Input: part model. Units: mm. Frame: model coordinates. Round coordinates to 2 decimals unless told otherwise and drop trailing zeros. Order: outer loops, then holes, each group sorted by start corner. A loop starts at its lowest first (then second) coordinate and runs counter-clockwise, first axis right, second up.
Item 1: Cut plane A-A on y = 4.3. Give the number of separate pieces and of enclosed holes in the cut face, then the cut area to 3 significant figures.
Item 2: Line query: L1, parallel to X at y = 3.5, z = -2.5 (3 decimals); L2, parallel to Y at x = 0, z = 1.75; L3, parallel to Y at x = 27, z = -3. Output: solid intervals per line, ascending.
Item 3: Cut plane D-D on x = 34.5. Output: boundary loops of the cut face in (y, z), then the cut area to 3 significant figures.
Item 4: First-contact query: pin 1 (1 mm diameter, centred on x = -6.5, z = 3.5, fed in from +Y); pin 2 (1.5 mm diameter, centred on x = -19, y = 3.5, fed in from -Z). Flat tips, straight axial feed; report the tip coordinate or a pass-through.
Item 5: Cut plane B-B on x = 9. Output: boundary loops of the cut face in (y, z), then the cut area to 3 significant figures.
Item 6: Cut plane C-C on z = 1.25. Output: boundary loops of the cut face in (x, y).
```python
from build123d import *

# Parameters (mm, degrees)
SKETCH1_W           = 43.1
SKETCH1_H           = 8
BOSS_EXTRUDE1_DEPTH = 2
SKETCH2_W           = 10
SKETCH2_H           = 2
BOSS_EXTRUDE2_DEPTH = 3
SKETCH3_W           = 33.1
SKETCH3_H           = 2
BOSS_EXTRUDE3_DEPTH = 1
CUT_EXTRUDE1_DEPTH  = 45.120403443


with BuildPart() as part:
    # Sketch1 → Boss-Extrude1 (new body)
    with BuildSketch(Plane(origin=(0, 0, 0), x_dir=(1, 0, 0), z_dir=(0, 1, 0))):
        with Locations((21.55, 0)):
            Rectangle(SKETCH1_W, SKETCH1_H)
    boss_extrude1 = extrude(amount=BOSS_EXTRUDE1_DEPTH)

    # Sketch2 → Boss-Extrude2 (add)
    with BuildSketch(Plane(origin=(0, 2, 0), x_dir=(1, 0, 0), z_dir=(0, 1, 0))):
        with Locations((38.1, -3)):
            Rectangle(SKETCH2_W, SKETCH2_H)
        with Locations((38.1, 3)):
            Rectangle(SKETCH2_W, SKETCH2_H)
    boss_extrude2 = extrude(amount=BOSS_EXTRUDE2_DEPTH)

    # Sketch3 → Boss-Extrude3 (add)
    with BuildSketch(Plane(origin=(0, 2, 0), x_dir=(1, 0, 0), z_dir=(0, 1, 0))):
        with Locations((16.55, -3)):
            Rectangle(SKETCH3_W, SKETCH3_H)
        with Locations((16.55, 3)):
            Rectangle(SKETCH3_W, SKETCH3_H)
    boss_extrude3 = extrude(amount=BOSS_EXTRUDE3_DEPTH)

    # Sketch4 → Cut-Extrude1 (cut, through all)
    with BuildSketch(Plane.XY.offset(4)):
        with BuildLine():
            Line((37.475, 3.5), (37.475, 5))
            Line((37.475, 5), (38.725, 5))
            Line((38.725, 5), (38.725, 3.5))
            ThreePointArc((38.725, 3.5), (38.1, 2.875), (37.475, 3.5))
        make_face()
    cut_extrude1 = extrude(amount=-CUT_EXTRUDE1_DEPTH, mode=Mode.SUBTRACT)

    # Mirror1: Boss-Extrude1, Boss-Extrude2, Boss-Extrude3, Cut-Extrude1 across plane
    add(boss_extrude1.mirror(Plane(origin=(0, 0, 0), x_dir=(0, 0, 1), z_dir=(1, 0, 0))))
    add(boss_extrude2.mirror(Plane(origin=(0, 0, 0), x_dir=(0, 0, 1), z_dir=(1, 0, 0))))
    add(boss_extrude3.mirror(Plane(origin=(0, 0, 0), x_dir=(0, 0, 1), z_dir=(1, 0, 0))))
    add(cut_extrude1.mirror(Plane(origin=(0, 0, 0), x_dir=(0, 0, 1), z_dir=(1, 0, 0))), mode=Mode.SUBTRACT)


solid = part.part
```
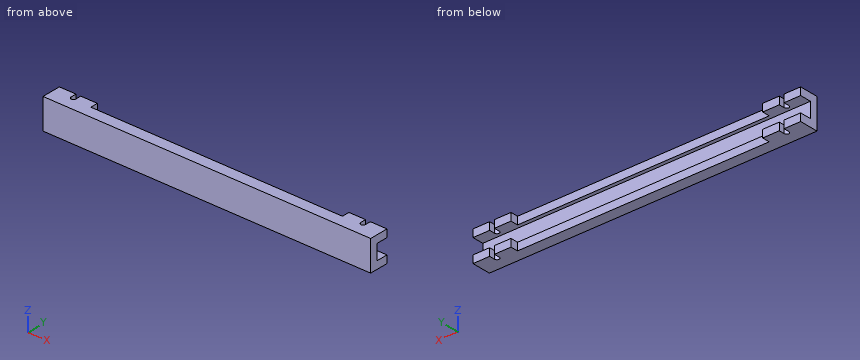
From the geometry:
1. separate pieces: 8
1. enclosed holes: 0
1. area: 70.0 mm2
2. L1: x = -43.1 to -38.725, -37.475 to -33.1, 33.1 to 37.475, 38.725 to 43.1
2. L2: y = 0 to 2
2. L3: y = 0 to 3
3. outline: (0, -4) - (5, -4) - (5, -2) - (2, -2) - (2, 2) - (5, 2) - (5, 4) - (0, 4) - close
3. area: 28.0 mm2
4. pin 1: stops at y = 3
4. pin 2: stops at z = -4
5. outline: (0, -4) - (3, -4) - (3, -2) - (2, -2) - (2, 2) - (3, 2) - (3, 4) - (0, 4) - close
5. area: 20.0 mm2
6. outline: (-43.1, 0) - (43.1, 0) - (43.1, 2) - (-43.1, 2) - close
